from build123d import *

# Parameters (mm, degrees)
SKETCH1_W                = 92
SKETCH1_H                = 12
BOSS_EXTRUDE1_DEPTH      = 51
SKETCH9_R                = 22
BOSS_EXTRUDE4_DEPTH      = 39
SKETCH9_W                = 25
SKETCH9_H                = 48
SKETCH9_W_2              = 8
SKETCH9_H_2              = 28
BOSS_EXTRUDE4_2_DEPTH    = 39
BOSS_EXTRUDE5_DEPTH      = 5
BOSS_EXTRUDE6_DEPTH      = 10
BOSS_EXTRUDE7_START      = -29
BOSS_EXTRUDE7_DEPTH      = 29
BOSS_EXTRUDE8_REACH      = 176.316
BOSS_EXTRUDE8_END_RADIUS = 22
SKETCH15_R               = 6
FILLET1_R                = 3
FILLET2_R                = 3
FILLET3_R                = 3
FILLET4_R                = 1
HOLE3_D                  = 12
HOLE3_DEPTH              = 12
LPATTERN1_COUNT          = 2
LPATTERN1_PITCH          = 44


# Read off the part's stored shape, not the designer's step: M6 Tapped Hole1
with BuildPart() as part:
    # Sketch1 → Boss-Extrude1 (new body)
    with BuildSketch(Plane.XY):
        with Locations((46, 6)):
            Rectangle(SKETCH1_W, SKETCH1_H)
    extrude(amount=BOSS_EXTRUDE1_DEPTH)



with BuildPart() as body_2:
    # Sketch9 → Boss-Extrude4 (new body)
    with BuildSketch(Plane.XY.offset(51)):
        with Locations((0, 114)):
            Circle(SKETCH9_R)
    extrude(amount=-BOSS_EXTRUDE4_DEPTH)


with BuildPart() as body_3:
    # Sketch9 → Boss-Extrude4 2 (new body)
    with BuildSketch(Plane.XY.offset(51)):
        with Locations((72, 112)):
            Rectangle(SKETCH9_W, SKETCH9_H)
        with Locations((72, 112)):
            Rectangle(SKETCH9_W_2, SKETCH9_H_2, mode=Mode.SUBTRACT)
    extrude(amount=-BOSS_EXTRUDE4_2_DEPTH)


with BuildPart() as part_1:
    add(part.part)

    add(body_2.part)  # Boss-Extrude5 merges body 2
    # Sketch10 → Boss-Extrude5 (add, symmetric)
    with BuildSketch(Plane.ZY):
        Polygon((0, 0), (0, 12), (12, 88), (12, 94), (51, 94), (51, 88), (51, 12), (51, 0), align=None)
    extrude(amount=BOSS_EXTRUDE5_DEPTH, both=True)

    # Sketch12 → Hole2 (revolve, cut)
    with BuildSketch(Plane(origin=(0, 114, 12), x_dir=(0, 1, 0), z_dir=(1, 0, 0))):
        Polygon((0, 0), (0, 39.001), (10, 39.001), (10, 5), (16, 5), (16, 0), align=None)
    revolve(axis=Axis((0, 114, 122), (0, 0, -1)), mode=Mode.SUBTRACT)


    add(body_3.part)  # Boss-Extrude6 merges body 3
    # Sketch13 → Boss-Extrude6 (add)
    with BuildSketch(Plane.XY.offset(51)):
        with BuildLine():
            Line((92, 12), (5, 12))
            Line((5, 12), (5, 92.575714714))
            ThreePointArc((5, 92.575714714), (21.85559741, 116.516517804), (0, 136))
            Line((0, 136), (59.5, 136))
            Line((59.5, 136), (59.5, 88))
            Line((59.5, 88), (84.5, 88))
            Line((84.5, 88), (92, 12))
        make_face()
    extrude(amount=-BOSS_EXTRUDE6_DEPTH)

    # Sketch14 → Boss-Extrude7 (add)
    with BuildSketch(Plane(origin=(0, 0, 12), x_dir=(-1, 0, 0), z_dir=(0, 0, -1)).offset(BOSS_EXTRUDE7_START)):
        with BuildLine():
            Line((-59.5, 119), (-59.5, 109))
            Line((-59.5, 109), (-21.424285286, 109))
            ThreePointArc((-21.424285286, 109), (-22, 114), (-21.424285286, 119))
            Line((-21.424285286, 119), (-59.5, 119))
        make_face()
    extrude(amount=BOSS_EXTRUDE7_DEPTH)

    # Boss-Extrude8: up to this cylinder (the profile starts outside it)
    boss_extrude8_end = Plane(origin=(0, 114, 28), z_dir=(0, 0, 1)) * Cylinder(BOSS_EXTRUDE8_END_RADIUS, 397.632, mode=Mode.PRIVATE)
    # Sketch15 → Boss-Extrude8 (add, up to the surface)
    with BuildSketch(Plane(origin=(0, 139, 0), x_dir=(1, 0, 0), z_dir=(0, 1, 0)), mode=Mode.PRIVATE) as boss_extrude8_sk1:
        with Locations(Location((0, -28, 0), (0, 0, 270))):
            Circle(SKETCH15_R)
    boss_extrude8_tool1 = extrude(boss_extrude8_sk1.sketch, amount=-BOSS_EXTRUDE8_REACH, mode=Mode.PRIVATE) - boss_extrude8_end
    add(boss_extrude8_tool1.solids().sort_by_distance((0, 139, 28))[0])

    # M6 Tapped Hole1 outline → M6 Tapped Hole1 (revolve, cut)
    with BuildSketch(Plane.XY.offset(28)):
        Polygon((0, 123.682411551), (2.5, 123.682411551), (2.5, 138.475), (3.025, 139), (0, 139), align=None)
    revolve(axis=Axis((0, 0, 28), (0, 1, 0)), mode=Mode.SUBTRACT)

    # Fillet1
    # the kernel refuses this fillet: 3 mm, written as the material it adds along each edge
    with BuildSketch(Plane(origin=(59.5, 136, 41), x_dir=(-1, 0, 0), z_dir=(0, -1, 0))) as fillet1_piece_1:
        with BuildLine():
            CenterArc((FILLET1_R, FILLET1_R), FILLET1_R, 180, 90)
            Line((0, FILLET1_R), (0, 0))
            Line((0, 0), (FILLET1_R, 0))
        make_face()
    extrude(amount=24.5)
    # the kernel refuses this fillet: 3 mm, written as the material it takes off along each edge
    with BuildSketch(Plane(origin=(59.5, 88, 41), x_dir=(0, 1, 0), z_dir=(0, 0, -1))) as fillet1_2_piece_1:
        with BuildLine():
            CenterArc((FILLET1_R, FILLET1_R), FILLET1_R, 180, 90)
            Line((0, FILLET1_R), (0, 0))
            Line((0, 0), (FILLET1_R, 0))
        make_face()
    extrude(amount=36.5, mode=Mode.SUBTRACT)
    # the kernel refuses this fillet: 3 mm, written as the material it takes off along each edge
    with BuildSketch(Plane(origin=(-7.5, 136, 41), x_dir=(0, 0, 1), z_dir=(1, 0, 0))) as fillet1_3_piece_1_section:
        with BuildLine():
            CenterArc((FILLET1_R, FILLET1_R), FILLET1_R, 180, 90)
            Line((0, FILLET1_R), (0, 0))
            Line((0, 0), (FILLET1_R, 0))
        make_face()
    fillet1_3_piece_1 = extrude(amount=64, mode=Mode.PRIVATE)
    fillet1_3_piece_1 = fillet1_3_piece_1 - Plane(origin=(0, 114, 41.685678885), x_dir=(1, 0, 0), z_dir=(0, 0, 1)) * Cylinder(22, 140, mode=Mode.PRIVATE)
    add(fillet1_3_piece_1, mode=Mode.SUBTRACT)
    with BuildSketch(Plane(origin=(59.5, 136, 38), x_dir=(1, 0, 0), z_dir=(0, 0, -1))) as fillet1_3_piece_2:
        with BuildLine():
            CenterArc((FILLET1_R, FILLET1_R), FILLET1_R, 180, 90)
            Line((0, FILLET1_R), (0, 0))
            Line((0, 0), (FILLET1_R, 0))
        make_face()
    extrude(amount=33.5, mode=Mode.SUBTRACT)
    with BuildSketch(Plane(origin=(56.5, 136, 38), x_dir=(0, 0, 1), z_dir=(-1, 0, 0))) as fillet1_3_piece_3:
        with BuildLine():
            CenterArc((3 + FILLET1_R, -FILLET1_R), FILLET1_R, 90, 90)
            Line((3, -FILLET1_R), (3, 0))
            Line((3, 0), (3 + FILLET1_R, 0))
        make_face()
    revolve(axis=Axis((56.5, 136, 38), (0, 1, 0)), revolution_arc=90, mode=Mode.SUBTRACT)

    # Fillet2
    fillet2_edges = [part_1.edges().sort_by_distance(p)[0] for p in [
        (68, 98, 31.5),
        (76, 98, 31.5),
        (76, 126, 31.5),
        (68, 126, 31.5),
    ]]
    fillet(fillet2_edges, radius=FILLET2_R)

    # Fillet3
    # the kernel refuses this fillet: 3 mm, written as the material it takes off along each edge
    with BuildSketch(Plane(origin=(84.5, 136, 58.5), x_dir=(-1, 0, 0), z_dir=(0, 0, -1))) as fillet3_piece_1:
        with BuildLine():
            CenterArc((FILLET3_R, -FILLET3_R), FILLET3_R, 90, 90)
            Line((0, -FILLET3_R), (0, 0))
            Line((0, 0), (FILLET3_R, 0))
        make_face()
    extrude(amount=54, mode=Mode.SUBTRACT)
    with BuildSketch(Plane(origin=(84.5, 88, 41), x_dir=(0, 1, 0), z_dir=(0, 0, -1))) as fillet3_piece_2:
        with BuildLine():
            CenterArc((FILLET3_R, -FILLET3_R), FILLET3_R, 90, 90)
            Line((0, -FILLET3_R), (0, 0))
            Line((0, 0), (FILLET3_R, 0))
        make_face()
    extrude(amount=36.5, mode=Mode.SUBTRACT)

    # Fillet4
    fillet4_edges = [part_1.edges().sort_by_distance(p)[0] for p in [
        (1e-09, 135.999999999, 21.999999993),
    ]]
    fillet(fillet4_edges, radius=FILLET4_R)

    # Hole3
    with Locations(Plane(origin=(0, 12, 0), x_dir=(1, 0, 0), z_dir=(0, 1, 0))):
        with Locations((73, -12)):
            hole3 = Hole(HOLE3_D / 2, depth=HOLE3_DEPTH)

    # LPattern1: Hole3 ×2
    with Locations(*[(-i * LPATTERN1_PITCH, 0, 0) for i in range(1, LPATTERN1_COUNT)]):
        add(hole3, mode=Mode.SUBTRACT)


solid = part_1.part
Could you check a few things on this model? Use its own coordinates, in mm. A direction names the side the tool comes from. Give positions to 0.01 mm unless a question says otherwise; leave off trailing zeros. Write each loop counter-clockwise with the first axis right and the second up, starting at its lowest first coordinate (ties: lowest second). Pieces come first, ordered by that corner, then holes. Notation, with made-up numbers: (74, 29) - (103, 29) arc R26 ccw to (103, 54) - close; hole circle Ø1 at (-27, 38.25). An arc over 180 degrees is marked (long way). Use CSV: the item, a comma, the result in double quotes. Start each with the question number.
Item 1: I'm going to push flat-ended pins straight in: pin 1 (12.5 mm diameter, centred on x = 52, z = 11, fed in from +Y); pin 2 (12.5 mm diameter, centred on y = 68, z = 17, fed in from +X); pin 3 (19.5 mm diameter, centred on x = 20.5, z = 39, fed in from +Y); pin 4 (6 mm diameter, centred on x = -8.5, y = 48, fed in from -Z). Where does each tip first touch, or does it pass through?
Item 2: For faces 5 (the face through (15.43, 98.32, 26.7)), 6 (the face through (0, 138, 22)), 7 (the face through (40, 119, 27)), 8 (the face through (75.14, 125.1, 31.23)), which set-ups out of +Z, -Z, +X, -X, +Y, -Y let a thin tool reach every point of the face, with its end or its side?
Item 3: If we mould it in two halves opening along X, with no side actions, what happens to faces 1 (the face through (84.5, 110, 32)), 2 (the face through (-9.736, 101.303, 14.465)), 3 (the face through (60.4, 88.86, 26.7)), 4 (the face through (43, 0, 25))? For each: pulls with the +X half, pulls with the -X half, needs draft (parallel to the pull), parting line crosses it, or undercut.
Item 4: I want a section at A-A, the plane x = 29. Please give me the cut outline in (y, z), then the cut area to 3 significant figures.
Item 5: I want a section at C-C, the plane y = 115. Please give me the cut outline in (x, z).
Item 6: I want a section at B-B, the plane x = 53.5. Please give me the cut outline in (y, z), then the cut area to 3 significant figures.
Item 7: If I drill on line 1 along X through (y, z) = (114, 13.1); line 2 along Y through (x, z) = (45.5, 39.5); line 3 along X through (y, z) = (127.5, 28), over which ranges is the centre line in solid material (lowest first)?
Item 8: I want a section at D-D, the plane z = 14. Give the number of separate pieces and of enclosed holes in the cut face, then the cut area to 3 significant figures.
Findings:
1,pin 1,"stops at y = 119"
1,pin 2,"stops at x = 5"
1,pin 3,"stops at y = 136"
1,pin 4,"passes through"
2,face 5,"-Z"
2,face 6,"+Y"
2,face 7,"-Z, +Y"
2,face 8,"+Z, -Z"
3,face 1,"pulls with the +X half"
3,face 2,"undercut"
3,face 3,"undercut"
3,face 4,"needs draft"
4,outline,"(0, 0) - (12, 0) - (12, 6) - (0, 6) - close; (0, 18) - (12, 18) - (12, 41) - (109, 41) - (109, 12) - (119, 12) - (119, 41) - (133, 41) arc R3 ccw to (136, 44) - (136, 51) - (0, 51) - close"
4,area,"2,000 mm2"
5,outline,"(-21.98, 12) - (-15.97, 12) - (-15.97, 17) - (-9.95, 17) - (-9.95, 51) - (-21.98, 51) - close; (9.95, 17) - (15.97, 17) - (15.97, 12) - (68, 12) - (68, 51) - (9.95, 51) - close; (76, 12) - (84.5, 12) - (84.5, 51) - (76, 51) - close"
6,outline,"(0, 0) - (12, 0) - (12, 41) - (109, 41) - (109, 12) - (119, 12) - (119, 41) - (133, 41) arc R3 ccw to (136, 44) - (136, 51) - (0, 51) - close"
6,area,"2,140 mm2"
7,line 1,"x = -22 to -16, 16 to 68, 76 to 84.5"
7,line 2,"y = 0 to 12, 109 to 119"
7,line 3,"x = -17.37 to -2.5, 2.5 to 17.37, 59.5 to 84.5"
8,separate pieces,"3"
8,enclosed holes,"2"
8,area,"3,760 mm2"
